```python
from build123d import *

# Parameters (mm, degrees)
SKETCH001_W  = 6
SKETCH001_H  = 6
PAD001_DEPTH = 0.1
FILLET001_R  = 0.3
PAD008_DEPTH = 0.7
FILLET003_R  = 0.29
PAD009_DEPTH = 0.7
FILLET004_R  = 0.29
PAD010_DEPTH = 0.7
FILLET005_R  = 0.29
SKETCH_W     = 6
SKETCH_H     = 6
PAD_DEPTH    = 3.5
FILLET_R     = 0.3
SKETCH004_R  = 0.5
PAD003_DEPTH = 0.6
SKETCH003_R  = 0.5
PAD004_DEPTH = 0.6
SKETCH005_R  = 0.5
PAD002_DEPTH = 0.6
SKETCH002_R  = 0.5
PAD005_DEPTH = 0.6
SKETCH006_R  = 1.75
PAD006_DEPTH = 9.5
FILLET006_R  = 0.1
PAD007_DEPTH = 0.7
FILLET002_R  = 0.29


with BuildPart() as fillet001:
    # Sketch001 → Pad001 (new body)
    with BuildSketch(Plane.XY.offset(3.5)):
        with Locations((3.15, -2.25)):
            Rectangle(SKETCH001_W, SKETCH001_H)
    extrude(amount=PAD001_DEPTH)

    # Fillet001
    fillet001_edges = [fillet001.edges().sort_by_distance(p)[0] for p in [
        (6.15, -5.25, 3.55),
        (0.15, -5.25, 3.55),
        (6.15, 0.75, 3.55),
        (0.15, 0.75, 3.55),
    ]]
    fillet(fillet001_edges, radius=FILLET001_R)


with BuildPart() as fillet003:
    # Sketch008 → Pad008 (new body)
    with BuildSketch(Plane.XZ.offset(0.35)):
        Polygon((-0.15, 1.5), (0.15, 1.5), (0.15, -0.5), (-0.15, -1.5), (0.15, -2.5), (0.15, -3.5), (-0.15, -3.5), (-0.15, -2.5), (-0.45, -1.5), (-0.15, -0.5), align=None)
    extrude(amount=-PAD008_DEPTH)

    # Fillet003
    fillet003_edges = [fillet003.edges().sort_by_distance(p)[0] for p in [
        (-0.15, 0, -2.5),
        (-0.15, 0, -0.5),
        (-0.45, 0, -1.5),
        (-0.15, 0, 1.5),
        (0.15, 0, -0.5),
        (-0.15, 0, -1.5),
        (0.15, 0, -2.5),
    ]]
    fillet(fillet003_edges, radius=FILLET003_R)


with BuildPart() as fillet004:
    # Sketch009 → Pad009 (new body)
    with BuildSketch(Plane.XZ.offset(4.85)):
        Polygon((6.45, 1.5), (6.15, 1.5), (6.15, -0.5), (6.45, -1.5), (6.15, -2.5), (6.15, -3.5), (6.45, -3.5), (6.45, -2.5), (6.75, -1.5), (6.45, -0.5), align=None)
    extrude(amount=-PAD009_DEPTH)

    # Fillet004
    fillet004_edges = [fillet004.edges().sort_by_distance(p)[0] for p in [
        (6.45, -4.5, -2.5),
        (6.45, -4.5, -0.5),
        (6.75, -4.5, -1.5),
        (6.45, -4.5, 1.5),
        (6.15, -4.5, -0.5),
        (6.45, -4.5, -1.5),
        (6.15, -4.5, -2.5),
    ]]
    fillet(fillet004_edges, radius=FILLET004_R)


with BuildPart() as fillet005:
    # Sketch010 → Pad010 (new body)
    with BuildSketch(Plane.XZ.offset(0.35)):
        Polygon((6.45, 1.5), (6.15, 1.5), (6.15, -0.5), (6.45, -1.5), (6.15, -2.5), (6.15, -3.5), (6.45, -3.5), (6.45, -2.5), (6.75, -1.5), (6.45, -0.5), align=None)
    extrude(amount=-PAD010_DEPTH)

    # Fillet005
    fillet005_edges = [fillet005.edges().sort_by_distance(p)[0] for p in [
        (6.45, 0, -2.5),
        (6.45, 0, -0.5),
        (6.75, 0, -1.5),
        (6.45, 0, 1.5),
        (6.15, 0, -0.5),
        (6.45, 0, -1.5),
        (6.15, 0, -2.5),
    ]]
    fillet(fillet005_edges, radius=FILLET005_R)


with BuildPart() as fillet_body:
    # Sketch → Pad (new body)
    with BuildSketch(Plane.XY):
        with Locations((3.15, -2.25)):
            Rectangle(SKETCH_W, SKETCH_H)
    extrude(amount=PAD_DEPTH)

    # Fillet
    fillet_edges = [fillet_body.edges().sort_by_distance(p)[0] for p in [
        (6.15, 0.75, 1.75),
        (6.15, -5.25, 1.75),
        (0.15, -5.25, 1.75),
        (0.15, 0.75, 1.75),
    ]]
    fillet(fillet_edges, radius=FILLET_R)


with BuildPart() as pad003:
    # Pad003 base: copy of Fillet body
    add(fillet_body.part)

    # Sketch004 → Pad003 (new body)
    with BuildSketch(Plane.XY.offset(3.5)):
        with Locations((5.15, -0.25)):
            Circle(SKETCH004_R)
    extrude(amount=PAD003_DEPTH)


with BuildPart() as pad004:
    # Pad004 base: copy of Fillet body
    add(fillet_body.part)

    # Sketch003 → Pad004 (new body)
    with BuildSketch(Plane.XY.offset(3.5)):
        with Locations((5.15, -4.25)):
            Circle(SKETCH003_R)
    extrude(amount=PAD004_DEPTH)


with BuildPart() as pad002:
    # Pad002 base: copy of Fillet body
    add(fillet_body.part)

    # Sketch005 → Pad002 (new body)
    with BuildSketch(Plane.XY.offset(3.5)):
        with Locations((1.15, -0.25)):
            Circle(SKETCH005_R)
    extrude(amount=PAD002_DEPTH)


with BuildPart() as pad005:
    # Pad005 base: copy of Fillet body
    add(fillet_body.part)

    # Sketch002 → Pad005 (new body)
    with BuildSketch(Plane.XY.offset(3.5)):
        with Locations((1.15, -4.25)):
            Circle(SKETCH002_R)
    extrude(amount=PAD005_DEPTH)


with BuildPart() as fillet006:
    # Pad006 base: copy of Fillet body
    add(fillet_body.part)

    # Sketch006 → Pad006 (new body)
    with BuildSketch(Plane.XY.offset(3.5)):
        with Locations((3.15, -2.25)):
            Circle(SKETCH006_R)
    extrude(amount=PAD006_DEPTH)

    # Fillet006
    fillet006_edges = [fillet006.edges().sort_by_distance(p)[0] for p in [
        (1.4, -2.25, 13),
    ]]
    fillet(fillet006_edges, radius=FILLET006_R)


with BuildPart() as obj1:
    # Sketch007 → Pad007 (new body)
    with BuildSketch(Plane.XZ.offset(4.85)):
        Polygon((-0.15, 1.5), (0.15, 1.5), (0.15, -0.5), (-0.15, -1.5), (0.15, -2.5), (0.15, -3.5), (-0.15, -3.5), (-0.15, -2.5), (-0.45, -1.5), (-0.15, -0.5), align=None)
    extrude(amount=-PAD007_DEPTH)

    # Fillet002
    fillet002_edges = [obj1.edges().sort_by_distance(p)[0] for p in [
        (-0.15, -4.5, -2.5),
        (-0.15, -4.5, -0.5),
        (-0.45, -4.5, -1.5),
        (-0.15, -4.5, 1.5),
        (0.15, -4.5, -0.5),
        (-0.15, -4.5, -1.5),
        (0.15, -4.5, -2.5),
    ]]
    fillet(fillet002_edges, radius=FILLET002_R)

    add(fillet001.part)
    add(fillet003.part)
    add(fillet004.part)
    add(fillet005.part)
    add(pad003.part)
    add(pad004.part)
    add(pad002.part)
    add(pad005.part)
    add(fillet006.part)


solid = obj1.part
```
CAD build for the part. Positions are in the model's coordinates, mm. A direction names the side the tool comes from. Round coordinates to 2 decimals unless told otherwise and drop trailing zeros. Order: outer loops, then holes, each group sorted by start corner. A loop starts at its lowest first (then second) coordinate and runs counter-clockwise, first axis right, second up.
Q1. Wall check: L1, parallel to Z at x = 2.5, y = -3.6; L2, parallel to Y at x = 2.25, z = 7; L3, parallel to X at y = -1.85, z = 0.5. Give the ranges that are in metal, low to high.
Q2. Which spindle directions (+Z, -Z, +X, -X, +Y, -Y) get a long thin tool onto all of the face, cutting with end or side? Do faces 1 (the flat face through (1, 0, 4.1)), 2 (the flat face through (1.8, -0.9, 3.6)), 3 (the flat face through (3, -2, 0)). Say none if no direction does.
Q3. Slice it at B-B (y = -2.25). Write the cut outline in (x, z).
Q4. Drop flat-ended pins along their axis: pin 1 (0.8 mm diameter, centred on y = -4.5, z = -3, fed in from -X); pin 2 (0.8 mm diameter, centred on x = 1.5, y = -0.5, fed in from +Z); pin 3 (0.8 mm diameter, centred on y = 0, z = -3, fed in from +X). Give the stop position or say it passes through.
Q5. Slice it at A-A (x = 1.15). Write the cut outline in (y, z), and give its area (3 significant figures).
Q6. Two-plate mould, pull along Y, no slides. Class faces 4 (the flat face through (6.15, -2, 2)), 5 (the flat face through (3, -2, 13)), 6 (the flat face through (3, 0.75, 2)): pulls with the +Y half, pulls with the -Y half, needs draft (parallel to the pull), parting line crosses it, or undercut.
Q7. Slice it at C-C (z = 3). Write the cut outline in (x, y), and give its area (3 significant figures).
Q8. Slice it at D-D (x = 3.15). Write the cut outline in (y, z).
Results below:
1. L1: z = 0 to 13
1. L2: y = -3.75 to -0.75
1. L3: x = 0.15 to 6.15
2. face 1: +Z, -X, +Y
2. face 2: +Z
2. face 3: -Z, +Y, -Y
3. outline: (0.15, 0) - (6.15, 0) - (6.15, 3.6) - (4.9, 3.6) - (4.9, 12.9) arc R0.1 ccw to (4.8, 13) - (1.5, 13) arc R0.1 ccw to (1.4, 12.9) - (1.4, 3.6) - (0.15, 3.6) - close
4. pin 1: stops at x = -0.15
4. pin 2: stops at z = 4.1
4. pin 3: stops at x = 6.45
5. outline: (-5.25, 0) - (0.75, 0) - (0.75, 3.6) - (0.25, 3.6) - (0.25, 4.1) - (-0.75, 4.1) - (-0.75, 3.6) - (-3.75, 3.6) - (-3.75, 4.1) - (-4.75, 4.1) - (-4.75, 3.6) - (-5.25, 3.6) - close
5. area: 22.6 mm2
6. face 4: undercut
6. face 5: needs draft
6. face 6: pulls with the +Y half
7. outline: (0.15, -4.95) arc R0.3 ccw to (0.45, -5.25) - (5.85, -5.25) arc R0.3 ccw to (6.15, -4.95) - (6.15, 0.45) arc R0.3 ccw to (5.85, 0.75) - (0.45, 0.75) arc R0.3 ccw to (0.15, 0.45) - close
7. area: 35.9 mm2
8. outline: (-5.25, 0) - (0.75, 0) - (0.75, 3.6) - (-0.5, 3.6) - (-0.5, 12.9) arc R0.1 ccw to (-0.6, 13) - (-3.9, 13) arc R0.1 ccw to (-4, 12.9) - (-4, 3.6) - (-5.25, 3.6) - close
